Autodesk Inventor part; units mm, degrees
ref_plane "YZ Plane" through (0, 0, 0) normal (1, 0, 0) x (0, 1, 0)
ref_plane "XZ Plane" through (0, 0, 0) normal (0, 1, 0) x (-1, 0, 0)
ref_plane "XY Plane" through (0, 0, 0) normal (0, 0, 1) x (1, 0, 0)
sketch "Sketch1" plane through (0, 0, 0) normal (0, 0, 1) x (1, 0, 0)
  line L0 (35.093, -7.2202) -> (-19.907, -7.2202)
  line L1 (-19.907, -7.2202) -> (-19.907, 74.7798)
  line L2 (-19.907, 74.7798) -> (35.093, 74.7798)
  line L3 (35.093, 74.7798) -> (35.093, -7.2202)
  line L4 (-1.6316, 73.7798) -> (15.8684, 73.7798)
  line L5 (15.8684, 73.7798) -> (15.8684, 38.2798)
  line L6 (15.8684, 38.2798) -> (-1.6316, 38.2798)
  line L7 (-1.6316, 38.2798) -> (-1.6316, 73.7798)
  circle A0 centre (7.5885, 28.2798) radius 5.75
  line L8 (12.233, 6.0025) -> (3.233, 6.0025)
  line L9 (3.233, 6.0025) -> (3.233, -3.9975)
  line L10 (3.233, -3.9975) -> (12.233, -3.9975)
  line L11 (12.233, -3.9975) -> (12.233, 6.0025)
  circle A1 centre (7.5885, 28.2798) radius 1.25
  line L12 (3.233, 6.0025) -> (-2.767, 6.0025)
  line L13 (-2.767, 6.0025) -> (-2.767, -3.9975)
  line L14 (-2.767, -3.9975) -> (3.233, -3.9975)
  line L15 (3.233, -3.9975) -> (3.233, 6.0025)
  line L16 (12.233, 5.3167) -> (16.7288, 5.3167)
  line L17 (16.7288, 5.3167) -> (16.7288, 2.7767)
  line L18 (16.7288, 2.7767) -> (12.233, 2.7767)
  line L19 (12.233, 2.7767) -> (12.233, 5.3167)
  line L20 (12.233, -1.5375) -> (12.233, 1.0025)
  line L21 (12.233, -3.4895) -> (12.233, -0.9495)
  line L22 (12.233, 2.2687) -> (16.7288, 2.2687)
  line L23 (16.7288, 2.2687) -> (16.7288, -0.2713)
  line L24 (16.7288, -0.2713) -> (12.233, -0.2713)
  line L25 (12.233, -0.2713) -> (12.233, 2.2687)
  line L26 (12.233, -0.7793) -> (16.7288, -0.7793)
  line L27 (16.7288, -0.7793) -> (16.7288, -3.3193)
  line L28 (16.7288, -3.3193) -> (12.233, -3.3193)
  line L29 (12.233, -3.3193) -> (12.233, -0.7793)
  circle A2 centre (0.233, 0.9987) radius 1.5
  circle A3 centre (0.3684, 66.2798) radius 0.75
  circle A4 centre (0.3684, 63.7398) radius 0.75
  circle A5 centre (0.3684, 61.1998) radius 0.75
  circle A6 centre (0.3684, 58.6598) radius 0.75
  circle A7 centre (0.3684, 56.1198) radius 0.75
  circle A8 centre (0.3684, 53.5798) radius 0.75
  circle A9 centre (0.3684, 51.0398) radius 0.75
  circle A10 centre (0.3684, 48.4998) radius 0.75
  circle A11 centre (13.8684, 63.7398) radius 0.75
  circle A12 centre (13.8684, 58.6598) radius 0.75
  circle A13 centre (13.8684, 56.1198) radius 0.75
  circle A14 centre (13.8684, 53.5798) radius 0.75
  circle A15 centre (13.8684, 48.4998) radius 0.75
  circle A16 centre (13.8684, 66.2798) radius 0.75
  circle A17 centre (13.8684, 51.0398) radius 0.75
  circle A18 centre (13.8684, 61.1998) radius 0.75
  line L30 (-17.907, 69.7798) -> (-16.407, 69.7798)
  line L31 (-16.407, 69.7798) -> (-16.407, -2.2202)
  line L32 (-16.407, -2.2202) -> (-17.907, -2.2202)
  line L33 (-17.907, -2.2202) -> (-17.907, 69.7798)
  line L34 (-15.367, -2.2202) -> (-13.867, -2.2202)
  line L35 (-13.867, -2.2202) -> (-13.867, 69.7798)
  line L36 (-13.867, 69.7798) -> (-15.367, 69.7798)
  line L37 (-15.367, 69.7798) -> (-15.367, -2.2202)
  line L38 (31.593, 69.7798) -> (33.093, 69.7798)
  line L39 (33.093, 69.7798) -> (33.093, -2.2202)
  line L40 (33.093, -2.2202) -> (31.593, -2.2202)
  line L41 (31.593, -2.2202) -> (31.593, 69.7798)
  line L42 (30.553, -2.2202) -> (29.053, -2.2202)
  line L43 (29.053, -2.2202) -> (29.053, 69.7798)
  line L44 (29.053, 69.7798) -> (30.553, 69.7798)
  line L45 (30.553, 69.7798) -> (30.553, -2.2202)
  line L46 (5.8684, 68.7798) -> (10.8684, 68.7798)
  line L47 (10.8684, 68.7798) -> (10.8684, 63.7798)
  line L48 (10.8684, 63.7798) -> (5.8684, 63.7798)
  line L49 (5.8684, 63.7798) -> (5.8684, 68.7798)
  line L50 (6.8684, 55.8198) -> (10.8684, 55.8198)
  line L51 (10.8684, 55.8198) -> (10.8684, 53.2798)
  line L52 (10.8684, 53.2798) -> (6.8684, 53.2798)
  line L53 (6.8684, 53.2798) -> (6.8684, 55.8198)
  line L54 (5.8684, 48.2798) -> (10.8684, 48.2798)
  line L55 (10.8684, 48.2798) -> (10.8684, 43.2798)
  line L56 (10.8684, 43.2798) -> (5.8684, 43.2798)
  line L57 (5.8684, 43.2798) -> (5.8684, 48.2798)
  circle A19 centre (0.8684, 71.2798) radius 1.5
  circle A20 centre (0.8684, 40.7798) radius 1.5
  point P0 (0, 0)
  point P1 (0, 0)
  dimension "d0" = 82
  dimension "d1" = 55
  dimension "d2" = 17.5
  dimension "d3" = 35.5
  dimension "d4" = 11.5
  dimension "d5" = 2.5
  dimension "d6" = 1
  dimension "d7" = 10
  dimension "d8" = 27.4955
  dimension "d9" = 9
  dimension "d10" = 10
  dimension "d11" = 6
  dimension "d12" = 22.86
  dimension "d13" = 19.2246
  dimension "d14" = 2.54
  dimension "d15" = 0.6858
  dimension "d16" = 10
  dimension "d17" = 2.54
  dimension "d18" = 0.508
  dimension "d19" = 4.4958
  dimension "d20" = 4.4958
  dimension "d21" = 2.54
  dimension "d22" = 4.4958
  dimension "d23" = 0.508
  dimension "d24" = 3
  dimension "d25" = 1.5
  dimension "d26" = 7.5
  dimension "d27" = 2
  dimension "d28" = 1.5
  dimension "d29" = 1.5
  dimension "d30" = 1.5
  dimension "d31" = 1.5
  dimension "d32" = 1.5
  dimension "d33" = 1.5
  dimension "d34" = 1.5
  dimension "d35" = 2.54
  dimension "d36" = 2.54
  dimension "d37" = 2.54
  dimension "d38" = 2.54
  dimension "d39" = 2.54
  dimension "d40" = 2.54
  dimension "d41" = 2.54
  dimension "d42" = 1.5
  dimension "d43" = 1.5
  dimension "d44" = 1.5
  dimension "d45" = 1.5
  dimension "d46" = 1.5
  dimension "d47" = 1.5
  dimension "d48" = 1.5
  dimension "d49" = 1.5
  dimension "d50" = 2.54
  dimension "d51" = 2.54
  dimension "d52" = 2.54
  dimension "d53" = 2.54
  dimension "d54" = 2.54
  dimension "d55" = 2.54
  dimension "d56" = 2.54
  dimension "d57" = 2
  dimension "d58" = 7.5
  dimension "d59" = 2
  dimension "d60" = 2
  dimension "d61" = 2
  dimension "d62" = 2
  dimension "d63" = 2
extrude "Extrusion1" add sketch "Sketch1" against normal blind 9 contours L0 L1 L2 L3 | L4 L5 L6 L7 | A0 | L11 L10 L9 L8 | L9 L14 L13 L12 | L16 L17 L18 L11 | L22 L23 L24 L11 | L11 L26 L27 L28 | A1 | A2 | A3 | A4 | A5 | A6 | A7 | A8 | A9 | A10 | A11 | A12 | A13 | A14 | A15 | A16 | A17 | A18 | L30 L31 L32 L33 | L37 L36 L35 L34 | L38 L39 L40 L41 | L42 L43 L44 L45 | L46 L47 L48 L49 | L50 L51 L52 L53 | L54 L55 L56 L57 | A19 | A20
extrude "Extrusion2" cut sketch "Sketch1" against normal blind 8 contours L30 L31 L32 L33 | L37 L36 L35 L34 | L38 L39 L40 L41 | L42 L43 L44 L45
fillet "Fillet1" radius 0.127 16 edges at (-13.867, 33.7798, 0) (-14.617, 69.7798, 0) (-15.367, 33.7798, 0) (-16.407, 33.7798, 0) (-17.157, 69.7798, 0) (-17.907, 33.7798, 0) (-14.617, -2.2202, 0) (-17.157, -2.2202, 0) (29.803, -2.2202, 0) (32.343, -2.2202, 0) (33.093, 33.7798, 0) (31.593, 33.7798, 0) (30.553, 33.7798, 0) (29.053, 33.7798, 0) (32.343, 69.7798, 0) (29.803, 69.7798, 0)
fillet "Fillet2" radius 0.508 4 edges at (7.593, 74.7798, 0) (35.093, 33.7798, 0) (7.593, -7.2202, 0) (-19.907, 33.7798, 0)
properties part number "Breadboard"
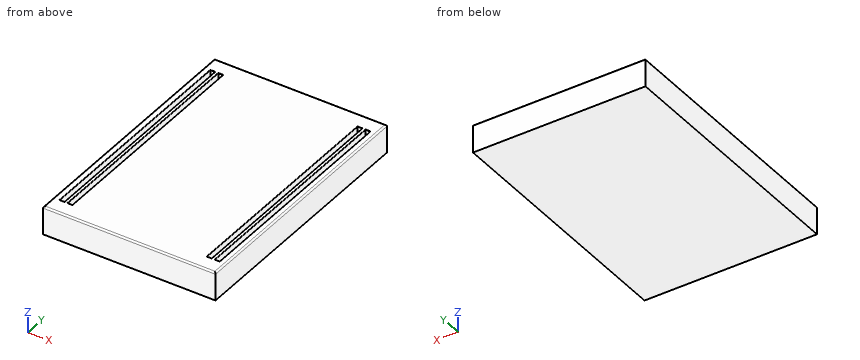
The model under review builds one solid part; all positions refer to its coordinate system, in mm. Give positions to 0.01 mm unless a question says otherwise; leave off trailing zeros. Loops run counter-clockwise (first coordinate to the right, second up) from the corner with the lowest first, then second, coordinate; pieces in that order, holes last. Notation, with made-up numbers: (59, 47.25) -> (106, 47.25) arc R25 cw to (106, 75.25) -> close; hole circle Ø7 at (10.25, 17). An arc over 180 degrees is marked (long way). Write each question's results on one line, items separated by ' | '.
1) Insertion check: pin 1 Ø0.8 at (x, y) = (32.5, 33) entering from +Z. The pin has a flat end and moves straight along its axis. Give the tip position at first contact, or say it passes through.
Conclusion:
pin 1: stops at z = -8
2) Take a section at A-A, the plane z = -4.5. Give the boundary of the cut face in (x, y).
Conclusion:
outline: (-19.91, -7.22) -> (35.09, -7.22) -> (35.09, 74.78) -> (-19.91, 74.78) -> close; hole (-17.91, -2.22) -> (-16.41, -2.22) -> (-16.41, 69.78) -> (-17.91, 69.78) -> close; hole (-15.37, -2.22) -> (-13.87, -2.22) -> (-13.87, 69.78) -> (-15.37, 69.78) -> close; hole (29.05, -2.22) -> (30.55, -2.22) -> (30.55, 69.78) -> (29.05, 69.78) -> close; hole (31.59, -2.22) -> (33.09, -2.22) -> (33.09, 69.78) -> (31.59, 69.78) -> close
3) For line 1 along X through (y, z) = (64, -6.5); line 2 along Y through (x, z) = (32, -7.25); line 3 along Y through (x, z) = (24, -0.25), list the stretches that pass through material, from the lowest coordinate up. Write a range as from..to.
Conclusion:
line 1: x = -19.91..-17.91, -16.41..-15.37, -13.87..29.05, 30.55..31.59, 33.09..35.09 | line 2: y = -7.22..-2.22, 69.78..74.78 | line 3: y = -7.15..74.71
